Autodesk Fusion 360 part; units mm, degrees
sketch "Sketch2" plane through (0, 0, 0) normal (0, 0, 1) x (1, 0, 0)
  circle A0 centre (-70, 0) radius 17
  arc A1 (65, 20) -> (65, -20) centre (89.1778, 0) ccw
  line L0 (65, -20) -> (102, -20)
  line L1 (65, 19.9864) -> (102.1, 19.9864)
  line L2 (102.1, 19.9864) -> (102.1, -20)
  line L3 (102.1, -20) -> (65, -20)
  arc A2 (102.1, 19.9864) -> (55, 25) centre (78.4273, 21.3408) ccw
  arc A3 (55, -25) -> (102.1, -20) centre (78.427, -21.3413) ccw
  line L4 (55, 25) -> (-75, 25)
  line L5 (-75, 25) -> (-75, -25)
  line L6 (-75, -25) -> (55, -25)
  arc A4 (-75, 25) -> (-75, -25) centre (-75, 0) ccw
  point P0 (100, -20)
  point P1 (100, 20)
  point P2 (57.8, 0.0068)
  point P3 (55, 25)
  point P4 (55, -25)
  dimension "d3" = 34
sketch "Sketch3" plane through (0, 0, 0) normal (0, 0, 1) x (1, 0, 0)
  line L0 (65, 20) -> (102.1, 20)
  line L1 (102.1, 20) -> (102.1, -20)
  line L2 (102.1, -20) -> (65, -20)
  line L3 (65, -20) -> (65, 20)
  line L4 (65, 20) -> (65, -20)
  arc A0 (65, 20) -> (65, -20) centre (89.1778, 0) ccw
extrude "Extrude1" add sketch "Sketch2" along normal blind 10 contours A0 L2 A2 A3 L4 L5 L6 | A0 L5 A4
extrude "Extrude2" cut sketch "Sketch3" along normal blind 10
Can you work these out from the model? Positions are in its coordinate system, mm. A direction names the side the tool comes from. Give positions to 0.01 mm unless a question says otherwise; leave off trailing zeros. Order: outer loops, then holes, each group sorted by start corner. A loop starts at its lowest first (then second) coordinate and runs counter-clockwise, first axis right, second up. Notation, with made-up numbers: M -17,-38.75 L 39,-38.75 A18 cw 39,-11.75 Z; hole C 86,71.25 d3. An arc over 180 degrees is marked long. Use a Markdown table: item, result. Add a question column.
Item 1: Suppose I cut it at D-D (x = -18.5). List the corners of the cut face in (y, z) for me, then the cut area to 3 significant figures.
Item 2: Will these pins go through, and if not, where does the flat tip stop? pin 1 (1 mm diameter, centred on y = 26, z = 3.5, fed in from +X); pin 2 (3 mm diameter, centred on x = 83, z = 5, fed in from -Y); pin 3 (1.5 mm diameter, centred on x = -29, z = 9, fed in from -Y); pin 4 (2 mm diameter, centred on x = -13.5, y = 15, fed in from -Z).
Item 3: For faces 1 (the flat face through (-9, 25, 5)), 2 (the flat face through (84, -20, 5)), 3 (the flat face through (-11, -25, 5)), 4 (the flat face through (0, 1, 0)), which set-ups out of +Z, -Z, +X, -X, +Y, -Y let a thin tool reach every point of the face, with its end or its side?
Item 4: We'd pull the mould along Y, two halves only. Please class faces 5 (the flat face through (0, 1, 10)), 6 (the cylindrical face through (-99.994, -0.55, 4.93)), 7 (the cylindrical face through (-82.53, -11.49, 4.93)): +Y half, -Y half, draft (parallel to the pull), parting line (faces both ways), or undercut.
Item 5: Suppose I cut it at C-C (y = 0). List the corners of the cut face in (x, z) for me.
Item 6: Suppose I cut it at A-A (x = -70). List the corners of the cut face in (y, z) for me, then the cut area to 3 significant figures.
Item 7: If I drill on L1, parallel to Y at x = -70, z = 4; L2, parallel to Y at x = -15.5, z = 4.5; L3, parallel to Y at x = 91, z = 7, over which ranges is the centre line in solid material (lowest first)? Write a range as [from, to].
Answer sheet:
| question | item | result |
|---|---|---|
| 1 | outline | M -25,0 L 25,0 L 25,10 L -25,10 Z |
| 1 | area | 500 mm² |
| 2 | pin 1 | stops at x = 101.77 |
| 2 | pin 2 | stops at y = -44.85 |
| 2 | pin 3 | stops at y = -25 |
| 2 | pin 4 | stops at z = 0 |
| 3 | face 1 | +Z, -Z, -X, +Y |
| 3 | face 2 | +Z, -Z, +X |
| 3 | face 3 | +Z, -Z, -X, -Y |
| 3 | face 4 | -Z, +X, -X, +Y, -Y |
| 4 | face 5 | draft |
| 4 | face 6 | parting line |
| 4 | face 7 | undercut |
| 5 | outline | M -100,0 L -87,0 L -87,10 L -100,10 Z; M -53,0 L 57.8,0 L 57.8,10 L -53,10 Z |
| 6 | outline | M -25,0 L -17,0 L -17,10 L -25,10 Z; M 17,0 L 25,0 L 25,10 L 17,10 Z |
| 6 | area | 160 mm² |
| 7 | L1 | y = [-25, -17], [17, 25] |
| 7 | L2 | y = [-25, 25] |
| 7 | L3 | y = [-41.44, -20], [20, 41.44] |
